Design review of the part built by this model. Coordinates are the model's own, in mm. Give positions to 0.01 mm unless a question says otherwise; leave off trailing zeros. Write each loop counter-clockwise with the first axis right and the second up, starting at its lowest first coordinate (ties: lowest second). Pieces come first, ordered by that corner, then holes. Notation, with made-up numbers: (31, -29) -> (76, -29) arc R18 cw to (76, -10) -> close; hole circle Ø7 at (54.25, -26.75). An arc over 180 degrees is marked (long way). Put each result on its own line as item: value. Start each with the question number.
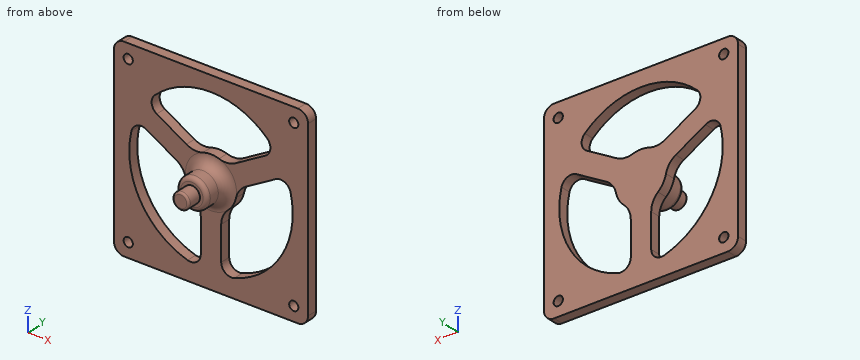
from build123d import *

# Parameters (mm, degrees)
SKETCH1_W                      = 95
SKETCH1_H                      = 95
BOSS_EXTRUDE1_DEPTH            = 5
FILLET1_R                      = 5
M4_CLEARANCE_HOLE1_D           = 4.5
M4_CLEARANCE_HOLE1_CSINK_D     = 4.55
M4_CLEARANCE_HOLE1_CSINK_ANGLE = 90
SKETCH5_R                      = 7.5
BOSS_EXTRUDE2_DEPTH            = 12
SKETCH6_R                      = 4
BOSS_EXTRUDE3_DEPTH            = 7
FILLET2_R                      = 2
FILLET3_R                      = 5
FILLET4_R                      = 1
CUT_EXTRUDE2_REACH             = 73.334
FILLET5_R                      = 5
FILLET6_R                      = 10


with BuildPart() as part:
    # Sketch1 → Boss-Extrude1 (new body)
    with BuildSketch(Plane(origin=(0, 0, 0), x_dir=(1, 0, 0), z_dir=(0, 1, 0))):
        Rectangle(SKETCH1_W, SKETCH1_H)
    extrude(amount=BOSS_EXTRUDE1_DEPTH)

    # Fillet1
    fillet1_edges = [part.edges().sort_by_distance(p)[0] for p in [
        (-47.50000000000001, 2.5, 47.5),
        (-47.50000000000001, 2.5, -47.5),
        (47.49999999999999, 2.5, -47.5),
        (47.49999999999999, 2.5, 47.5),
    ]]
    fillet(fillet1_edges, radius=FILLET1_R)

    # M4 Clearance Hole1 (through all)
    with Locations(Plane(origin=(-40.5, 5, -40.5), x_dir=(0, 0, 1), z_dir=(0, 1, 0))):
        with Locations((0, 0), (0, 81), (81, 81), (81, 0)):
            CounterSinkHole(M4_CLEARANCE_HOLE1_D / 2, M4_CLEARANCE_HOLE1_CSINK_D / 2, counter_sink_angle=M4_CLEARANCE_HOLE1_CSINK_ANGLE)

    # Sketch5 → Boss-Extrude2 (add)
    with BuildSketch(Plane.XZ):
        with Locations(Location((0, 0, 0), (0, 0, 90))):
            Circle(SKETCH5_R)
    extrude(amount=BOSS_EXTRUDE2_DEPTH)

    # Sketch6 → Boss-Extrude3 (add)
    with BuildSketch(Plane.XZ.offset(12)):
        with Locations(Location((0, 0, 0), (0, 0, 270))):
            Circle(SKETCH6_R)
    extrude(amount=BOSS_EXTRUDE3_DEPTH)

    # Fillet2
    fillet2_edges = [part.edges().sort_by_distance(p)[0] for p in [
        (-4.71e-15, -12, -7.5),
    ]]
    fillet(fillet2_edges, radius=FILLET2_R)

    # Fillet3
    fillet3_edges = [part.edges().sort_by_distance(p)[0] for p in [
        (-4.71e-15, 0, -7.5),
    ]]
    fillet(fillet3_edges, radius=FILLET3_R)

    # Fillet4
    fillet4_edges = [part.edges().sort_by_distance(p)[0] for p in [
        (1.22e-15, -19, 4),
    ]]
    fillet(fillet4_edges, radius=FILLET4_R)

    # Sketch2 → Cut-Extrude2 (cut, up to next)
    with BuildSketch(Plane(origin=(0, 5, 0), x_dir=(1, 0, 0), z_dir=(0, 1, 0)), mode=Mode.PRIVATE) as cut_extrude2_sk1:
        with BuildLine():
            Line((5.000000000000003, 39.68626966596886), (4.999999999999999, 11.456439237389601))
            ThreePointArc((4.999999999999999, 11.456439237389601), (10.8253175473055, 6.249999999999979), (12.421567416492215, -1.398092599772662))
            Line((12.421567416492215, -1.398092599772662), (36.86931771216872, -15.51300781406241))
            ThreePointArc((36.86931771216872, -15.51300781406241), (34.64101615137759, 19.99999999999991), (5.000000000000003, 39.68626966596886))
        make_face()
    cut_extrude2_tool1 = extrude(cut_extrude2_sk1.sketch, amount=-CUT_EXTRUDE2_REACH, mode=Mode.PRIVATE) & part.part
    # Sketch2 → Cut-Extrude2 (cut, up to next)
    with BuildSketch(Plane(origin=(0, 5, 0), x_dir=(1, 0, 0), z_dir=(0, 1, 0)), mode=Mode.PRIVATE) as cut_extrude2_sk2:
        with BuildLine():
            Line((-5.000000000000003, 39.68626966596886), (-4.999999999999999, 11.456439237389601))
            ThreePointArc((-4.999999999999999, 11.456439237389601), (-10.825317547305497, 6.249999999999976), (-12.42156741649221, -1.3980925997726692))
            Line((-12.42156741649221, -1.3980925997726692), (-36.86931771216872, -15.513007814062414))
            ThreePointArc((-36.86931771216872, -15.513007814062414), (-34.64101615137759, 19.999999999999922), (-5.000000000000003, 39.68626966596886))
        make_face()
    cut_extrude2_tool2 = extrude(cut_extrude2_sk2.sketch, amount=-CUT_EXTRUDE2_REACH, mode=Mode.PRIVATE) & part.part
    # Sketch2 → Cut-Extrude2 (cut, up to next)
    with BuildSketch(Plane(origin=(0, 5, 0), x_dir=(1, 0, 0), z_dir=(0, 1, 0)), mode=Mode.PRIVATE) as cut_extrude2_sk3:
        with BuildLine():
            Line((-7.4215674164921674, -10.058346637617028), (-31.86931771216868, -24.173261851906783))
            ThreePointArc((-31.86931771216868, -24.173261851906783), (2.45e-15, -40), (31.869317712168694, -24.173261851906773))
            Line((31.869317712168694, -24.173261851906773), (7.421567416492171, -10.058346637617028))
            ThreePointArc((7.421567416492171, -10.058346637617028), (7.7e-16, -12.5), (-7.4215674164921674, -10.058346637617028))
        make_face()
    cut_extrude2_tool3 = extrude(cut_extrude2_sk3.sketch, amount=-CUT_EXTRUDE2_REACH, mode=Mode.PRIVATE) & part.part
    add(cut_extrude2_tool1.solids().sort_by_distance((22.174901, 5, -12.802685))[0], mode=Mode.SUBTRACT)
    add(cut_extrude2_tool2.solids().sort_by_distance((-22.174901, 5, -12.802685))[0], mode=Mode.SUBTRACT)
    add(cut_extrude2_tool3.solids().sort_by_distance((0, 5, 25.60537))[0], mode=Mode.SUBTRACT)

    # Fillet5
    fillet5_edges = [part.edges().sort_by_distance(p)[0] for p in [
        (-36.86931771216872, 2.5, 15.513007814062414),
        (-4.999999999999998, 2.5, -39.68626966596885),
        (31.869317712168694, 2.5, 24.173261851906776),
        (-31.869317712168684, 2.5, 24.173261851906787),
        (5.000000000000002, 2.5, -39.68626966596885),
        (36.86931771216872, 2.5, 15.51300781406241),
    ]]
    fillet(fillet5_edges, radius=FILLET5_R)

    # Fillet6
    fillet6_edges = [part.edges().sort_by_distance(p)[0] for p in [
        (-4.999999999999998, 2.5, -11.456439237389603),
        (-12.42156741649221, 2.5, 1.398092599772669),
        (-7.421567416492167, 2.5, 10.058346637617028),
        (7.42156741649217, 2.5, 10.058346637617026),
        (12.421567416492213, 2.5, 1.3980925997726628),
        (4.999999999999999, 2.5, -11.4564392373896),
    ]]
    fillet(fillet6_edges, radius=FILLET6_R)


solid = part.part
Q1. Take a section at C-C on y = 2.5. State how many separate pieces and enclosed holes the cut face has, then the cut area to 3 significant figures.
Q2. For pin 1 (1.5 mm diameter, centred on y = -4, z = 1.5, fed in from +X); pin 2 (10 mm diameter, centred on x = 1.5, y = -6.5, fed in from -Z); pin 3 (10 mm diameter, centred on x = -9, z = -15, fed in from -Y), all flat-tipped, find the tip position at first contact; note any pin that passes through.
Q3. Take a section at A-A on x = 0. Give the boundary of the cut face in (y, z).
Q4. To check wall thickness, follow probe 1 along Z at (x, y) = (-40.5, 2.4); probe 2 along X at (y, z) = (2.5, -15). State the ranges of each line that lie inside material, in increasing order. Write a range as from..to.
Q5. Take a section at B-B on z = -40.5. Give the boundary of the cut face in (x, y) (3 decimals).
Result:
1. separate pieces: 1
1. enclosed holes: 7
1. area: 5,310 mm^2
2. pin 1: stops at x = 7.7
2. pin 2: stops at z = -8.85
2. pin 3: stops at y = 0
3. outline: (-19, -3) arc R1 ccw to (-18, -4) -> (-12, -4) -> (-12, -5.5) arc R2 ccw to (-10, -7.5) -> (-5, -7.5) arc R5 cw to (0, -12.5) -> (0, -47.5) -> (5, -47.5) -> (5, 12.5) -> (0, 12.5) arc R5 cw to (-5, 7.5) -> (-10, 7.5) arc R2 ccw to (-12, 5.5) -> (-12, 4) -> (-18, 4) arc R1 ccw to (-19, 3) -> close; (0, 40) -> (5, 40) -> (5, 47.5) -> (0, 47.5) -> close
4. probe 1: z = -47.5..-42.75, -38.25..38.25, 42.75..47.5
4. probe 2: x = -47.5..-37.08, -5.16..5.16, 37.08..47.5
5. outline: (-47.5, 0) -> (-42.75, 0) -> (-42.75, 4.975) -> (-42.775, 5) -> (-47.5, 5) -> close; (-38.25, 0) -> (38.25, 0) -> (38.25, 4.975) -> (38.225, 5) -> (-38.225, 5) -> (-38.25, 4.975) -> close; (42.75, 0) -> (47.5, 0) -> (47.5, 5) -> (42.775, 5) -> (42.75, 4.975) -> close
